from build123d import *

# Parameters (mm, degrees)
BOSS_EXTRUDE1_DEPTH = 5.9
SKETCH2_R           = 1
CUT_EXTRUDE1_DEPTH  = 5.9
SKETCH3_W           = 4
SKETCH3_H           = 4
CUT_EXTRUDE2_DEPTH  = 1
SKETCH4_W           = 8
SKETCH4_H           = 5
BOSS_EXTRUDE2_DEPTH = 1.95


with BuildPart() as part:
    # Sketch1 → Boss-Extrude1 (new body)
    with BuildSketch(Plane(origin=(0, 0, 0), x_dir=(1, 0, 0), z_dir=(0, 1, 0))):
        with BuildLine():
            Line((-15, 6.5), (15, 6.5))
            ThreePointArc((15, 6.5), (21.5, 0), (15, -6.5))
            Line((15, -6.5), (-15, -6.5))
            ThreePointArc((-15, -6.5), (-21.5, 0), (-15, 6.5))
        make_face()
    extrude(amount=BOSS_EXTRUDE1_DEPTH)

    # Sketch2 → Cut-Extrude1 (cut)
    with BuildSketch(Plane(origin=(0, 5.9, 0), x_dir=(1, 0, 0), z_dir=(0, 1, 0))):
        with Locations(Location((-19, 0, 0), (0, 0, 270))):
            Circle(SKETCH2_R)
        with Locations(Location((19, 0, 0), (0, 0, 270))):
            Circle(SKETCH2_R)
    extrude(amount=-CUT_EXTRUDE1_DEPTH, mode=Mode.SUBTRACT)

    # Sketch3 → Cut-Extrude2 (cut)
    with BuildSketch(Plane(origin=(0, 5.9, 0), x_dir=(1, 0, 0), z_dir=(0, 1, 0))):
        Rectangle(SKETCH3_W, SKETCH3_H)
    extrude(amount=-CUT_EXTRUDE2_DEPTH, mode=Mode.SUBTRACT)

    # Sketch4 → Boss-Extrude2 (add)
    with BuildSketch(Plane.XZ):
        with Locations((9.93462309, 0.219446149)):
            Rectangle(SKETCH4_W, SKETCH4_H)
    extrude(amount=BOSS_EXTRUDE2_DEPTH)


solid = part.part
Can you work these out from the model? Positions are in its coordinate system, mm. A direction names the side the tool comes from. Give positions to 0.01 mm unless a question says otherwise; leave off trailing zeros. Write each loop counter-clockwise with the first axis right and the second up, starting at its lowest first coordinate (ties: lowest second). Pieces come first, ordered by that corner, then holes. Notation, with made-up numbers: (31, -27.75) -> (73, -27.75) arc R18 cw to (73, -5.75) -> close; hole circle Ø1 at (-12, -31.5). An arc over 180 degrees is marked (long way). Answer as a JSON object with one key per item and string values. Group by question number.
Item 1: We'd pull the mould along Z, two halves only. Please class faces 1 (the face through (0, 5.4, 2)), 2 (the face through (0, 3, -6.5)), 3 (the face through (0, 3, 6.5)), 4 (the face through (2, 5.4, 0)): +Z half, -Z half, draft (parallel to the pull), parting line (faces both ways), or undercut.
Item 2: For faces 5 (the face through (10, -1, -2.281)), 6 (the face through (0, 4.9, 0)), 7 (the face through (10, -1, 2.719)), 8 (the face through (5.935, -1, 0)), 9 (the face through (13.935, -1, 0)), which set-ups out of +Z, -Z, +X, -X, +Y, -Y let a thin tool reach every point of the face, with its end or its side?
Item 3: Suppose I cut it at C-C (y = 3.25). Please give me the cut outline in (x, z).
Item 4: Suppose I cut it at D-D (x = -5). Please give me the cut outline in (y, z), plus the area to 3 significant figures.
Item 5: Suppose I cut it at A-A (z = 0). Please give me the cut outline in (x, y), plus the area to 3 significant figures.
Item 6: Suppose I cut it at B-B (x = -19). Please give me the cut outline in (y, z), plus the area to 3 significant figures.
Item 7: Please list where these lines run through material, in increasing order: line 1 (X direction, y = 4.15, z = 0); line 2 (X direction, y = 1.75, z = -0.75); line 3 (Y direction, x = 16.5, z = -4.75). Write a range as [from, to].
Item 8: I'm going to push flat-ended pins straight in: P1, Ø1, axis at y = -1, z = 1.5, coming from the +X side; P2, Ø2.5, axis at x = 19, z = 0, coming from the -Y side; P3, Ø1.6, axis at y = -1, z = -1, coming from the -X side; P4, Ø1.8, axis at x = -19, z = 0, coming from the +Y side. Where does each tip first touch, or does it pass through?
Findings:
{
 "1": {"face 1": "undercut", "face 2": "-Z half", "face 3": "+Z half", "face 4": "undercut"},
 "2": {"face 5": "-Z, +X, -X, -Y", "face 6": "+Y", "face 7": "+Z, +X, -X, -Y", "face 8": "+Z, -Z, -X, -Y", "face 9": "+Z, -Z, +X, -Y"},
 "3": {"outline": "(-15, -6.5) -> (15, -6.5) arc R6.5 ccw to (15, 6.5) -> (-15, 6.5) arc R6.5 ccw to start; hole circle Ø2 at (-19, 0); hole circle Ø2 at (19, 0)"},
 "4": {"outline": "(0, -6.5) -> (5.9, -6.5) -> (5.9, 6.5) -> (0, 6.5) -> close", "area": "76.7 mm²"},
 "5": {"outline": "(-21.5, 0) -> (-20, 0) -> (-20, 5.9) -> (-21.5, 5.9) -> close; (-18, 0) -> (5.93, 0) -> (5.93, -1.95) -> (13.93, -1.95) -> (13.93, 0) -> (18, 0) -> (18, 5.9) -> (2, 5.9) -> (2, 4.9) -> (-2, 4.9) -> (-2, 5.9) -> (-18, 5.9) -> close; (20, 0) -> (21.5, 0) -> (21.5, 5.9) -> (20, 5.9) -> close", "area": "242 mm²"},
 "6": {"outline": "(0, -5.12) -> (5.9, -5.12) -> (5.9, -1) -> (0, -1) -> close; (0, 1) -> (5.9, 1) -> (5.9, 5.12) -> (0, 5.12) -> close", "area": "48.7 mm²"},
 "7": {"line 1": "x = [-21.5, -20], [-18, 18], [20, 21.5]", "line 2": "x = [-21.46, -19.66], [-18.34, 18.34], [19.66, 21.46]", "line 3": "y = [0, 5.9]"},
 "8": {"P1": "stops at x = 13.93", "P2": "stops at y = 0", "P3": "stops at x = 5.93", "P4": "passes through"}
}
